Can you work these out from the model? Positions are in its coordinate system, mm. Give positions to 0.01 mm unless a question says otherwise; leave off trailing zeros. Loops run counter-clockwise (first coordinate to the right, second up) from the corner with the lowest first, then second, coordinate; pieces in that order, holes last.
from build123d import *

# Parameters (mm, degrees)
F1_DEPTH = 3


with BuildPart() as f1:
    # F0 (on Front) → F1 (new body)
    with BuildSketch(Plane.XZ):
        Polygon((-157, -30), (157, -30), (157, -18), (160, -18), (160, -6), (157, -6), (157, 6), (160, 6), (160, 18), (157, 18), (157, 27), (144.761905, 27), (144.761905, 30), (129.52381, 30), (129.52381, 27), (114.285714, 27), (114.285714, 30), (99.047619, 30), (99.047619, 27), (83.809524, 27), (83.809524, 30), (68.571429, 30), (68.571429, 27), (53.333333, 27), (53.333333, 30), (38.095238, 30), (38.095238, 27), (22.857143, 27), (22.857143, 30), (7.619048, 30), (7.619048, 27), (-7.619048, 27), (-7.619048, 30), (-22.857143, 30), (-22.857143, 27), (-38.095238, 27), (-38.095238, 30), (-53.333333, 30), (-53.333333, 27), (-68.571429, 27), (-68.571429, 30), (-83.809524, 30), (-83.809524, 27), (-99.047619, 27), (-99.047619, 30), (-114.285714, 30), (-114.285714, 27), (-129.52381, 27), (-129.52381, 30), (-144.761905, 30), (-144.761905, 27), (-157, 27), (-157, 18), (-160, 18), (-160, 6), (-157, 6), (-157, -6), (-160, -6), (-160, -18), (-157, -18), align=None)
    extrude(amount=F1_DEPTH)


solid = f1.part
(1) Suppose I cut it at B-B on x = 90. List the corners of the cut face in (y, z) for me.
Returned:
outline: (-3, -30) - (0, -30) - (0, 27) - (-3, 27) - close
(2) Please list where these lines run through material, in increasing order: probe 1 along Z at (x, y) = (129, -2.4); probe 2 along X at (y, z) = (-2.8, -3.5).
Returned:
probe 1: z = -30 to 27
probe 2: x = -157 to 157
(3) Will these pins go through, and if not, where does the flat tip stop? P1, Ø0.9, axis at y = -1.5, z = 28.5, coming from the -X side; P2, Ø0.9, axis at x = -159, y = -2, coming from the +Z side; P3, Ø1.5, axis at x = 91, y = -1.5, coming from the +Z side.
Returned:
P1: stops at x = -144.76
P2: stops at z = 18
P3: stops at z = 27
(4) Suppose I cut it at A-A on z = -23.5. List the corners of the cut face in (x, y) for me, plus the area to 3 significant figures.
Returned:
outline: (-157, -3) - (157, -3) - (157, 0) - (-157, 0) - close
area: 942 mm2
